The listing builds one solid part. Answer for the finished solid, in the listing's coordinates (mm). A direction names the side the tool comes from. Give positions to 0.01 mm unless a question says otherwise; leave off trailing zeros. Write each loop counter-clockwise with the first axis right and the second up, starting at its lowest first coordinate (ties: lowest second). Pieces come first, ordered by that corner, then holes. Notation, with made-up numbers: (45, 1) - (97, 1) arc R6 ccw to (97, 11) - close; hole circle Ø7 at (-31, 41). An arc over 180 degrees is marked (long way). Answer as CSV lines item,"result". Start each with the question number.
(1) For a pull along Y with two mould halves and no side action, classify faces 1 (the face through (7.4, 4.5, 12.4)), 2 (the face through (7.012, 13.718, 3.268)), 3 (the face through (7.4, 0, 7.6)) as pulls with the +Y half, pulls with the -Y half, needs draft (parallel to the pull), parting line crosses it, or undercut.
(2) For faces 4 (the face through (6, 14, 4.5)), 5 (the face through (9, 8, 2)), 6 (the face through (0, 6, 4)), determine the directions among +Z, -Z, +X, -X, +Y, -Y from which every point of the face is accessible in a straight line to the end or side of a thin tool.
(3) Find section D-D (z = 1.5). Write down the section's boundary in (x, y).
(4) Straight lines are drawn through the part: probe 1 along Y at (x, z) = (7.5, 0.6); probe 2 along X at (y, z) = (10, 1.25). For each, find the intervals that lie inside material, in ascending order.
(5) Find section A-A (z = 10). Write down the section's boundary in (x, y).
(6) Find section B-B (x = 7.5). Write down the section's boundary in (y, z), then the cut area to 4 significant figures.
(7) Each of these flat-tipped pins is pushed along its axis until it touches: pin 1 Ø1.5 at (x, z) = (7, 10) entering from -Y; pin 2 Ø6 at (x, y) = (8.5, 11.5) entering from +Z; pin 3 Ø5.5 at (x, z) = (9, 10) entering from +Y; pin 4 Ø1 at (y, z) = (10, 2) entering from -X. Where does it stop, or does it pass through?
(8) Find section C-C (y = 10). Write down the section's boundary in (x, z), then the cut area to 4 significant figures.
from build123d import *

# Parameters (mm, degrees)
SKETCH_W        = 15
SKETCH_H        = 15.5
SKETCH_R        = 2.25
PAD_DEPTH       = 4.5
SKETCH001_R     = 3.75
POCKET_DEPTH    = 2.5
SKETCH002_W     = 15
SKETCH002_H     = 4.5
PAD001_DEPTH    = 11
SKETCH003_R     = 2.25
POCKET001_DEPTH = 6.5


with BuildPart() as part:
    # Sketch → Pad (new body)
    with BuildSketch(Plane.XY):
        with Locations((7.5, 7.75)):
            Rectangle(SKETCH_W, SKETCH_H)
        with Locations((7.5, 10)):
            Circle(SKETCH_R, mode=Mode.SUBTRACT)
    extrude(amount=PAD_DEPTH)

    # Sketch001 (on Face7 of Pad) → Pocket (cut)
    with BuildSketch(Plane.XY.offset(4.5)):
        with Locations((7.5, 10)):
            Circle(SKETCH001_R)
    extrude(amount=-POCKET_DEPTH, mode=Mode.SUBTRACT)

    # Sketch002 (on Face5 of Pocket) → Pad001 (join)
    with BuildSketch(Plane.XY.offset(4.5)):
        with Locations((7.5, 2.25)):
            Rectangle(SKETCH002_W, SKETCH002_H)
    extrude(amount=PAD001_DEPTH)

    # Sketch003 (on Face5 of Pad001) → Pocket001 (cut)
    with BuildSketch(Plane(origin=(0, 4.5, 0), x_dir=(-1, 0, 0), z_dir=(0, 1, 0))):
        with Locations((-7.5, 10)):
            Circle(SKETCH003_R)
    extrude(amount=-POCKET001_DEPTH, mode=Mode.SUBTRACT)


solid = part.part
Result set:
1,face 1,"pulls with the +Y half"
1,face 2,"undercut"
1,face 3,"pulls with the -Y half"
2,face 4,"+Z, +X, -X, +Y"
2,face 5,"+Z"
2,face 6,"+Z, -Z, -X, +Y, -Y"
3,outline,"(0, 0) - (15, 0) - (15, 15.5) - (0, 15.5) - close; hole circle Ø4.5 at (7.5, 10)"
4,probe 1,"0 to 7.75, 12.25 to 15.5"
4,probe 2,"0 to 5.25, 9.75 to 15"
5,outline,"(0, 0) - (5.25, 0) - (5.25, 4.5) - (0, 4.5) - close; (9.75, 0) - (15, 0) - (15, 4.5) - (9.75, 4.5) - close"
6,outline,"(0, 0) - (7.75, 0) - (7.75, 2) - (6.25, 2) - (6.25, 4.5) - (4.5, 4.5) - (4.5, 7.75) - (0, 7.75) - close; (0, 12.25) - (4.5, 12.25) - (4.5, 15.5) - (0, 15.5) - close; (12.25, 0) - (15.5, 0) - (15.5, 4.5) - (13.75, 4.5) - (13.75, 2) - (12.25, 2) - close"
6,area,"71.25 mm^2"
7,pin 1,"through"
7,pin 2,"z = 4.5"
7,pin 3,"y = 4.5"
7,pin 4,"x = 0"
8,outline,"(0, 0) - (5.25, 0) - (5.25, 2) - (3.75, 2) - (3.75, 4.5) - (0, 4.5) - close; (9.75, 0) - (15, 0) - (15, 4.5) - (11.25, 4.5) - (11.25, 2) - (9.75, 2) - close"
8,area,"39.75 mm^2"
